For this review, take the finished solid that the model builds, in its own axes (mm). A direction names the side the tool comes from. Coordinates: 2 decimals unless noted, no trailing zeros. Write each loop counter-clockwise with the first axis right and the second up, starting at its lowest first coordinate (ties: lowest second). Pieces come first, ordered by that corner, then holes. Notation, with made-up numbers: M 56.25,12 L 108.25,12 A18 cw 108.25,40 Z; hole C 32.5,1 d3. An arc over 180 degrees is marked long. One line per question, with ' | ' between items.
from build123d import *

# Parameters (mm, degrees)
SKETCH_1_W        = 13.075
SKETCH_1_H        = 14
SKETCH_1_R        = 1.25
EXTRUDE_2_DEPTH   = 2.9
SKETCH_1_W_2      = 12.871097853
EXTRUDE_2_2_DEPTH = 2.9
EXTRUDE_3_DEPTH   = 0.9


with BuildPart() as part:
    # Sketch 1 → Extrude 2 (new body)
    with BuildSketch(Plane(origin=(0, 0, 0), x_dir=(1, 0, 0), z_dir=(0, 1, 0))):
        with Locations((-7.968432469, -1.549350884)):
            Rectangle(SKETCH_1_W, SKETCH_1_H)
        with Locations(Location((-11.705932469, 3.250649116, 0), (0, 0, 270))):
            Circle(SKETCH_1_R, mode=Mode.SUBTRACT)
    extrude(amount=EXTRUDE_2_DEPTH)



with BuildPart() as body_2:
    # Sketch 1 → Extrude 2 2 (new body)
    with BuildSketch(Plane(origin=(0, 0, 0), x_dir=(1, 0, 0), z_dir=(0, 1, 0))):
        with Locations((21.408518604, -1.549350884)):
            Rectangle(SKETCH_1_W_2, SKETCH_1_H)
        with Locations(Location((25.044067531, 3.250649116, 0), (0, 0, 270))):
            Circle(SKETCH_1_R, mode=Mode.SUBTRACT)
    extrude(amount=EXTRUDE_2_2_DEPTH)


with BuildPart() as part_1:
    add(part.part)

    add(body_2.part)  # Extrude 3 merges body 2
    # Sketch 1_4 → Extrude 3 (add)
    with BuildSketch(Plane(origin=(0, 0, 0), x_dir=(1, 0, 0), z_dir=(0, 1, 0))):
        Polygon((14.769067531, 5.450649116), (6.669067531, 5.450649116), (-1.430932469, 5.450649116), (-1.430932469, -8.549350884), (14.972969678, -8.549350884), (14.972969678, 5.450649116), align=None)
    extrude(amount=EXTRUDE_3_DEPTH)


solid = part_1.part
1) Machinability: for faces 4 (the flat face through (-8, 2.9, 1)), 5 (the flat face through (14.973, 2, 2)), which of the approach directions +Z, -Z, +X, -X, +Y, -Y give a long, thin tool a straight path to every point of the face, cutting with its end or side? Answer none if there is none.
Responses:
face 4: +Z, -Z, +X, -X, +Y | face 5: +Z, -Z, +Y
2) We need section B-B on y = 1.3. State the section outline as (x, z) points, then the cut area to 3 significant figures.
Responses:
outline: M -14.51,-5.45 L -1.43,-5.45 L -1.43,8.55 L -14.51,8.55 Z; M 14.97,-5.45 L 27.84,-5.45 L 27.84,8.55 L 14.97,8.55 Z; hole C -11.71,-3.25 d2.5; hole C 25.04,-3.25 d2.5 | area: 353 mm^2
3) We need section A-A on z = -3.75. State the section outline as (x, y) points.
Responses:
outline: M -14.51,0 L -12.85,0 L -12.85,2.9 L -14.51,2.9 Z; M -10.56,0 L 23.9,0 L 23.9,2.9 L 14.97,2.9 L 14.97,0.9 L -1.43,0.9 L -1.43,2.9 L -10.56,2.9 Z; M 26.19,0 L 27.84,0 L 27.84,2.9 L 26.19,2.9 Z
4) The part is to be moulded in two halves that separate along X. For faces 1 (the cylindrical face through (-10.65, 1.43, -2.58)), 2 (the flat face through (27.844, 1, 2)), 3 (the flat face through (7, 0.5, -5.451)), say which applies: +X half, -X half, draft (parallel to the pull), parting line (faces both ways), or undercut.
Responses:
face 1: undercut | face 2: +X half | face 3: draft
5) We need section C-C on x = -11. State the section outline as (y, z) points, then the cut area to 3 significant figures.
Responses:
outline: M 0,-5.45 L 2.9,-5.45 L 2.9,-4.28 L 0,-4.28 Z; M 0,-2.22 L 2.9,-2.22 L 2.9,8.55 L 0,8.55 Z | area: 34.6 mm^2
6) We need section D-D on z = 4.25. State the section outline as (x, y) points, then the cut area to 3 significant figures.
Responses:
outline: M -14.51,0 L 27.84,0 L 27.84,2.9 L 14.97,2.9 L 14.97,0.9 L -1.43,0.9 L -1.43,2.9 L -14.51,2.9 Z | area: 90.0 mm^2
7) Insertion check: pin 1 Ø1.5 at (x, z) = (11.5, 5) entering from +Y; pin 2 Ø1 at (x, y) = (12.5, 2.5) entering from -Z. Each pin has a flat end and moves straight along its axis. Give the tip position at first contact, or say it passes through.
Responses:
pin 1: y = 0.9 | pin 2: through
8) To check wall thickness, follow line 1 along X through (y, z) = (2.4, -1.5); line 2 along X through (y, z) = (2.7, -4); line 3 along Z through (x, y) = (25, 1.85). State the ranges of each line that lie inside material, in increasing order. Write a range as [from, to].
Responses:
line 1: [-14.51, -1.43], [14.97, 27.84] | line 2: [-14.51, -12.71], [-10.71, -1.43], [14.97, 24.04], [26.04, 27.84] | line 3: [-5.45, -4.5], [-2, 8.55]
